from build123d import *

# Parameters (mm, degrees)
BOSS_EXTRUDE1_START     = 50
BOSS_EXTRUDE1_DEPTH     = 3
BOSS_EXTRUDE2_DEPTH     = 3
CUT_EXTRUDE1_DEPTH      = 120.526409216
CUT_EXTRUDE1_DEPTH_BACK = 120.526409216
SKETCH2_R               = 1.5
SKETCH3_W               = 56
SKETCH3_H               = 20
BOSS_EXTRUDE4_DEPTH     = 3
SKETCH4_W               = 56
SKETCH4_H               = 20
BOSS_EXTRUDE5_DEPTH     = 3


with BuildPart() as part:
    # Sketch1 → Boss-Extrude1 (new body)
    with BuildSketch(Plane.XY.offset(BOSS_EXTRUDE1_START)):
        with BuildLine():
            Line((-10, 105.25), (10, 105.25))
            ThreePointArc((10, 105.25), (17.071067812, 102.321067812), (20, 95.25))
            Line((20, 95.25), (20, -95.25))
            ThreePointArc((20, -95.25), (17.071067812, -102.321067812), (10, -105.25))
            Line((10, -105.25), (-10, -105.25))
            ThreePointArc((-10, -105.25), (-17.071067812, -102.321067812), (-20, -95.25))
            Line((-20, -95.25), (-20, 95.25))
            ThreePointArc((-20, 95.25), (-17.071067812, 102.321067812), (-10, 105.25))
        make_face()
    extrude(amount=BOSS_EXTRUDE1_DEPTH)


with BuildPart() as body_2:
    # Sketch1_3 → Boss-Extrude2 (new body)
    with BuildSketch(Plane.XY):
        with BuildLine():
            Line((-10, 105.25), (10, 105.25))
            ThreePointArc((10, 105.25), (17.071067812, 102.321067812), (20, 95.25))
            Line((20, 95.25), (20, -95.25))
            ThreePointArc((20, -95.25), (17.071067812, -102.321067812), (10, -105.25))
            Line((10, -105.25), (-10, -105.25))
            ThreePointArc((-10, -105.25), (-17.071067812, -102.321067812), (-20, -95.25))
            Line((-20, -95.25), (-20, 95.25))
            ThreePointArc((-20, 95.25), (-17.071067812, 102.321067812), (-10, 105.25))
        make_face()
    extrude(amount=-BOSS_EXTRUDE2_DEPTH)


with BuildPart() as cut_extrude1_tool:
    # Sketch2 → Cut-Extrude1 (new, two sides: drawn at the far end of the back side and taken through both)
    with BuildSketch(Plane.XY.offset(-CUT_EXTRUDE1_DEPTH_BACK)):
        with Locations((0, 95.25)):
            Circle(SKETCH2_R)
        with Locations(Location((0, -95.25, 0), (0, 0, 180))):
            Circle(SKETCH2_R)
    extrude(amount=CUT_EXTRUDE1_DEPTH + CUT_EXTRUDE1_DEPTH_BACK)


with BuildPart() as part_1:
    add(part.part)

    # Cut-Extrude1: cut by cut_extrude1_tool
    add(cut_extrude1_tool.part, mode=Mode.SUBTRACT)



with BuildPart() as body_2_1:
    add(body_2.part)

    # Cut-Extrude1: cut by cut_extrude1_tool
    add(cut_extrude1_tool.part, mode=Mode.SUBTRACT)


with BuildPart() as part_2:
    add(part_1.part)

    add(body_2_1.part)  # Boss-Extrude4 merges body 2
    # Sketch3 → Boss-Extrude4 (add)
    with BuildSketch(Plane.ZY.offset(20)):
        with Locations((25, 80.25)):
            Rectangle(SKETCH3_W, SKETCH3_H)
        with Locations((25, 40.25)):
            Rectangle(SKETCH3_W, SKETCH3_H)
        with Locations((25, 0.25)):
            Rectangle(SKETCH3_W, SKETCH3_H)
        with Locations((25, -39.75)):
            Rectangle(SKETCH3_W, SKETCH3_H)
        with Locations((25, -79.75)):
            Rectangle(SKETCH3_W, SKETCH3_H)
    extrude(amount=BOSS_EXTRUDE4_DEPTH)

    # Sketch4 → Boss-Extrude5 (add)
    with BuildSketch(Plane(origin=(20, 0, 0), x_dir=(0, 0, -1), z_dir=(1, 0, 0))):
        with Locations((-25, -79.75)):
            Rectangle(SKETCH4_W, SKETCH4_H)
        with Locations((-25, -39.75)):
            Rectangle(SKETCH4_W, SKETCH4_H)
    extrude(amount=BOSS_EXTRUDE5_DEPTH)


solid = part_2.part
Model file for the job. Use its own axes, mm. A direction names the side the tool comes from. Round coordinates to 2 decimals unless told otherwise and drop trailing zeros. Loops run counter-clockwise (first coordinate to the right, second up) from the corner with the lowest first, then second, coordinate; pieces in that order, holes last. Notation, with made-up numbers: (-1.5, 84.25) - (24.5, 84.25) arc R22 ccw to (24.5, 104.25) - close; hole circle Ø6 at (57, 34.25). An arc over 180 degrees is marked (long way). Write each question's results on one line, items separated by ' | '.
(1) Pin check, flat tips, straight feed: pin 1 (0.9 mm diameter, centred on y = 21, z = 52, fed in from -X); pin 2 (2.5 mm diameter, centred on x = 0, y = -95.25, fed in from +Z); pin 3 (10 mm diameter, centred on x = 16, z = 18, fed in from +Y); pin 4 (1.5 mm diameter, centred on x = -22, z = 22, fed in from -Y). Stop position of each tip, or through.
Answer below:
pin 1: stops at x = -20 | pin 2: passes through | pin 3: stops at y = -29.75 | pin 4: stops at y = -89.75
(2) Saw through at A-A, the plane z = 12. List the corners of the cut face in (x, y).
Answer below:
outline: (-23, -89.75) - (-20, -89.75) - (-20, -69.75) - (-23, -69.75) - close; (-23, -49.75) - (-20, -49.75) - (-20, -29.75) - (-23, -29.75) - close; (-23, -9.75) - (-20, -9.75) - (-20, 10.25) - (-23, 10.25) - close; (-23, 30.25) - (-20, 30.25) - (-20, 50.25) - (-23, 50.25) - close; (-23, 70.25) - (-20, 70.25) - (-20, 90.25) - (-23, 90.25) - close; (20, -89.75) - (23, -89.75) - (23, -69.75) - (20, -69.75) - close; (20, -49.75) - (23, -49.75) - (23, -29.75) - (20, -29.75) - close
(3) Saw through at B-B, the plane y = 36. List the corners of the cut face in (x, z).
Answer below:
outline: (-23, -3) - (20, -3) - (20, 0) - (-20, 0) - (-20, 50) - (20, 50) - (20, 53) - (-23, 53) - close
(4) 3-axis set-ups, long thin cutter, end or side, ignore diameter. For faces 1 (the flat face through (-20, -40, 25)), 2 (the flat face through (-20, 40, 25)), 3 (the flat face through (0, -1, 53)): which of +Z, -Z, +X, -X, +Y, -Y reach the whole face in a straight line?
Answer below:
face 1: +Y, -Y | face 2: +X, +Y, -Y | face 3: +Z, +X, -X, +Y, -Y
(5) Wall check: L1, parallel to Y at x = 0, z = -2; L2, parallel to Z at x = -11, y = -40; L3, parallel to X at y = 95.25, z = 51.2. Give the ranges that are in metal, low to high.
Answer below:
L1: y = -105.25 to -96.75, -93.75 to 93.75, 96.75 to 105.25 | L2: z = -3 to 0, 50 to 53 | L3: x = -20 to -1.5, 1.5 to 20
